```python
from build123d import *

# Parameters (mm, degrees)
SKETCH_1_W          = 30
SKETCH_1_H          = 30
EXTRUDE_1_DEPTH     = 10
CUT_EXTRUDE_1_DEPTH = 44.588989435
SKETCH_3_R          = 1
CUT_EXTRUDE_2_DEPTH = 3
SKETCH_4_W          = 10
SKETCH_4_H          = 10
EXTRUDE_2_DEPTH     = 10
SKETCH_5_R          = 1
EXTRUDE_3_DEPTH     = 1.6
SKETCH_6_R          = 2
EXTRUDE_4_DEPTH     = 6


with BuildPart() as part:
    # Эскиз1 → Бобышка-Вытянуть1 (new body)
    with BuildSketch(Plane(origin=(0, 0, 0), x_dir=(1, 0, 0), z_dir=(0, 1, 0))):
        with Locations((15, 15)):
            Rectangle(SKETCH_1_W, SKETCH_1_H)
    extrude(amount=EXTRUDE_1_DEPTH)

    # Эскиз2 → Вырез-Вытянуть1 (cut, through all)
    with BuildSketch(Plane.XY):
        Polygon((5, 0), (5, 4), (10, 4), (10, 6), (20, 6), (20, 4), (25, 4), (25, 0), align=None)
    extrude(amount=-CUT_EXTRUDE_1_DEPTH, mode=Mode.SUBTRACT)

    # Эскиз3 → Вырез-Вытянуть2 (cut)
    with BuildSketch(Plane(origin=(0, 10, 0), x_dir=(1, 0, 0), z_dir=(0, 1, 0))):
        with Locations(Location((3, 27, 0), (0, 0, 270))):
            Circle(SKETCH_3_R)
        with Locations(Location((15, 27, 0), (0, 0, 270))):
            Circle(SKETCH_3_R)
        with Locations(Location((27, 27, 0), (0, 0, 270))):
            Circle(SKETCH_3_R)
        with Locations(Location((27, 15, 0), (0, 0, 270))):
            Circle(SKETCH_3_R)
        with Locations(Location((27, 3, 0), (0, 0, 270))):
            Circle(SKETCH_3_R)
        with Locations(Location((15, 3, 0), (0, 0, 270))):
            Circle(SKETCH_3_R)
        with Locations(Location((3, 3, 0), (0, 0, 270))):
            Circle(SKETCH_3_R)
        with Locations(Location((3, 15, 0), (0, 0, 270))):
            Circle(SKETCH_3_R)
        with Locations(Location((15, 15, 0), (0, 0, 270))):
            Circle(SKETCH_3_R)
    extrude(amount=-CUT_EXTRUDE_2_DEPTH, mode=Mode.SUBTRACT)

    # Эскиз4 → Бобышка-Вытянуть2 (add)
    with BuildSketch(Plane(origin=(30, 0, 0), x_dir=(0, 0, -1), z_dir=(1, 0, 0))):
        with Locations((23, 5)):
            Rectangle(SKETCH_4_W, SKETCH_4_H)
    extrude(amount=EXTRUDE_2_DEPTH)

    # Эскиз5 → Бобышка-Вытянуть3 (add)
    with BuildSketch(Plane.ZY):
        with Locations(Location((-11.5, 6, 0), (0, 0, 180))):
            Circle(SKETCH_5_R)
    extrude(amount=EXTRUDE_3_DEPTH)

    # Эскиз6 → Бобышка-Вытянуть4 (add)
    with BuildSketch(Plane.ZY.offset(1.6)):
        with Locations((-11.5, 6)):
            Circle(SKETCH_6_R)
    extrude(amount=EXTRUDE_4_DEPTH)


solid = part.part
```
Input: part model. Units: mm. Frame: model coordinates. A direction names the side the tool comes from. Round coordinates to 2 decimals unless told otherwise and drop trailing zeros. Loops run counter-clockwise (first coordinate to the right, second up) from the corner with the lowest first, then second, coordinate; pieces in that order, holes last. Notation, with made-up numbers: (37, -37) - (56, -37) arc R25 ccw to (56, -19) - close; hole circle Ø10 at (-3.5, 65.5). An arc over 180 degrees is marked (long way). One line per item, written item: value. Start each with the question number.
(1) Contact query for flat-ended pins moving along their axis: P1, Ø2.5, axis at x = 15, z = -3, coming from the -Y side; P2, Ø5, axis at x = 34.5, y = 6.5, coming from the -Z side; P3, Ø1.6, axis at x = 27, z = -3, coming from the +Y side; P4, Ø2, axis at x = 34, z = -15.5, coming from the -Y side. Output: stop coordinate, or through.
(2) Section A-A, the plane z = -5.25. Return loops of the section in (x, y), plus the area to 3 significant figures.
(3) Section D-D, the plane z = -21.75. Return loops of the section in (x, y), plus the area to 3 significant figures.
(4) Ray query, line 1 (X direction, y = 7.7, z = -15); line 2 (X direction, y = 4.25, z = -16.5); line 3 (X direction, y = 5, z = -11). Return the intervals inside material, ascending. Write a range as [from, to].
(5) Draft query along Z for faces 1 (the cylindrical face through (14, 9, -27)), 2 (the flat face through (3, 7, -15)), 3 (the flat face through (40, 5, -23)), 4 (the flat face through (35, 5, -28)). Return one class per face: +Z half, -Z half, draft (parallel to the pull), parting line (faces both ways), or undercut.
(6) Access query for faces 5 (the flat face through (31, 0, -19)), 6 (the flat face through (15, 6, -15)), 7 (the flat face through (-1.6, 5.1, -10.6)), 8 (the cylindrical face through (3.676, 8.521, -27.737)). Directions: +Z, -Z, +X, -X, +Y, -Y. A direction counts if a zero-diameter tool reaches every point of the face in a straight line with its end or side. Return the directions, or none.
(7) Section C-C, the plane x = 15. Return loops of the section in (y, z), plus the area to 3 significant figures.
(8) Section B-B, the plane y = 5.5. Return loops of the section in (x, z).
Results below:
1. P1: y = 6
1. P2: z = -28
1. P3: y = 7
1. P4: through
2. outline: (0, 0) - (5, 0) - (5, 4) - (10, 4) - (10, 6) - (20, 6) - (20, 4) - (25, 4) - (25, 0) - (30, 0) - (30, 10) - (0, 10) - close
2. area: 200 mm^2
3. outline: (0, 0) - (5, 0) - (5, 4) - (10, 4) - (10, 6) - (20, 6) - (20, 4) - (25, 4) - (25, 0) - (40, 0) - (40, 10) - (0, 10) - close
3. area: 300 mm^2
4. line 1: [0, 2], [4, 14], [16, 26], [28, 30]
4. line 2: [0, 10], [20, 30]
4. line 3: [-7.6, -1.6], [0, 10], [20, 30]
5. face 1: undercut
5. face 2: undercut
5. face 3: draft
5. face 4: -Z half
6. face 5: +Z, -Z, +X, -X, -Y
6. face 6: +Z, -Z, -Y
6. face 7: none
6. face 8: +Y
7. outline: (6, -30) - (10, -30) - (10, -28) - (7, -28) - (7, -26) - (10, -26) - (10, -16) - (7, -16) - (7, -14) - (10, -14) - (10, -4) - (7, -4) - (7, -2) - (10, -2) - (10, 0) - (6, 0) - close
7. area: 102 mm^2
8. outline: (-7.6, -13.44) - (-1.6, -13.44) - (-1.6, -12.37) - (0, -12.37) - (0, -30) - (10, -30) - (10, 0) - (0, 0) - (0, -10.63) - (-1.6, -10.63) - (-1.6, -9.56) - (-7.6, -9.56) - close; (20, -30) - (30, -30) - (30, -28) - (40, -28) - (40, -18) - (30, -18) - (30, 0) - (20, 0) - close
